Geometry check sheet. Reference: the model listing, model coordinates, mm. Face numbers are marked on the shaded views. A direction names the side the tool comes from. Round coordinates to 2 decimals unless told otherwise and drop trailing zeros. Loops run counter-clockwise (first coordinate to the right, second up) from the corner with the lowest first, then second, coordinate; pieces in that order, holes last. Notation, with made-up numbers: M 41,41.5 L 73,41.5 A24 cw 73,56.5 Z; hole C -4,-30.75 d8. An arc over 180 degrees is marked long. Use one line per item in the form item = value. Start each with the question number.
1. Set-up check for the marked faces 4, 5, 6, 7 and 8: record each of +Z, -Z, +X, -X, +Y, -Y from which the full face is reachable in a straight line by a thin tool's end or side.
2. Cross-section at A-A (z = 27). Record the boundary of the cut face in (x, y), then the cut area to 3 significant figures.
3. Go/stop test with flat-tipped pins: pin 1 (12.5 mm diameter, centred on x = 0, y = -220, fed in from +Z); pin 2 (17.5 mm diameter, centred on x = 136, z = 13, fed in from -Y); pin 3 (6 mm diameter, centred on x = -20, y = -230, fed in from +Z); pin 4 (5 mm diameter, centred on x = 0.5, y = -229.5, fed in from +Z). Record where each tip stops, or that it passes through.
4. Cross-section at C-C (z = 8). Record the boundary of the cut face in (x, y).
5. Material ranges on line 1 (X direction, y = -250, z = 25.25); line 2 (Y direction, x = 0, z = 5.75); line 3 (X direction, y = -252.5, z = 26), recorded low to high.
6. Cross-section at D-D (y = -220). Record the boundary of the cut face in (x, z), then the cut area to 3 significant figures.
7. Cross-section at B-B (y = -250). Record the boundary of the cut face in (x, z).
8. Draft check along X on the marked faces 1, 2 and 3. Enter one of: pulls with the +X half, pulls with the -X half, needs draft (parallel to the pull), parting line crosses it, or undercut.
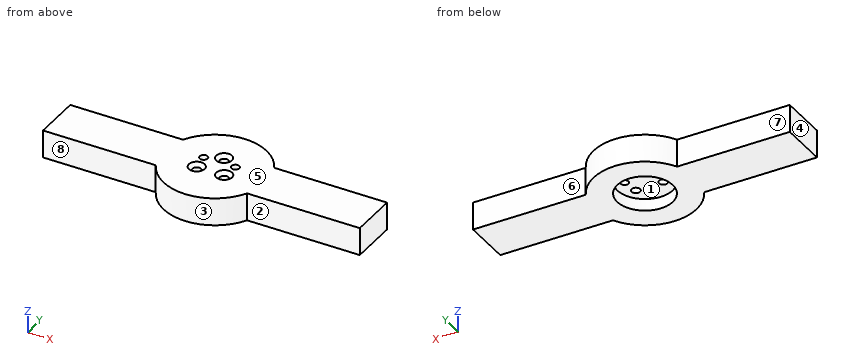
```python
from build123d import *

# Parameters (mm, degrees)
RESSALTO_EXTRUS_O1_DEPTH                             = 35
ESBO_O3_R                                            = 35
CORTE_EXTRUS_O2_DEPTH                                = 15
ESCAREADO_PARA_PARAFUSO_COM_CABE_A_ESCAR_D           = 11
ESCAREADO_PARA_PARAFUSO_COM_CABE_A_ESCAR_CSINK_D     = 20
ESCAREADO_PARA_PARAFUSO_COM_CABE_A_ESCAR_CSINK_ANGLE = 90
FUROS_GUIA_COM_10_0MM1_D                             = 10
ESBO_O2_R                                            = 35
CORTE_EXTRUS_O1_DEPTH                                = 15


with BuildPart() as part:
    # Esboço1 → Ressalto-extrusão1 (new body)
    with BuildSketch(Plane.XY):
        with BuildLine():
            Line((-200, -270), (-57.662812973, -270))
            ThreePointArc((-57.662812973, -270), (0, -305), (57.662812973, -270))
            Line((57.662812973, -270), (200, -270))
            Line((200, -270), (200, -210))
            Line((200, -210), (57.662812973, -210))
            ThreePointArc((57.662812973, -210), (0, -175), (-57.662812973, -210))
            Line((-57.662812973, -210), (-200, -210))
            Line((-200, -210), (-200, -270))
        make_face()
    extrude(amount=RESSALTO_EXTRUS_O1_DEPTH)

    # Esboço3 → Corte-extrusão2 (cut)
    with BuildSketch(Plane(origin=(0, 0, 0), x_dir=(-1, 0, 0), z_dir=(0, 0, -1))):
        with Locations((0, -240)):
            Circle(ESBO_O3_R)
    extrude(amount=-CORTE_EXTRUS_O2_DEPTH, mode=Mode.SUBTRACT)

    # Escareado para parafuso com cabeça escareada elevada de M101 (through all)
    with Locations(Plane.XY.offset(35)):
        with Locations((0, -220), (-17.320508076, -250), (17.320508076, -250)):
            CounterSinkHole(ESCAREADO_PARA_PARAFUSO_COM_CABE_A_ESCAR_D / 2, ESCAREADO_PARA_PARAFUSO_COM_CABE_A_ESCAR_CSINK_D / 2, counter_sink_angle=ESCAREADO_PARA_PARAFUSO_COM_CABE_A_ESCAR_CSINK_ANGLE)

    # Furos-guia com Ø10.0mm1 (through all)
    with Locations(Plane.XY.offset(35)):
        with Locations((-20, -230), (20, -230)):
            Hole(FUROS_GUIA_COM_10_0MM1_D / 2)

    # Esboço2 → Corte-extrusão1 (cut)
    with BuildSketch(Plane(origin=(0, 0, 0), x_dir=(-1, 0, 0), z_dir=(0, 0, -1))):
        with Locations((0, -240)):
            Circle(ESBO_O2_R)
    extrude(amount=-CORTE_EXTRUS_O1_DEPTH, mode=Mode.SUBTRACT)


solid = part.part
```
Reported:
q1.face_4 = +Z, -Z, -X, +Y, -Y
q1.face_5 = +Z, +X, -X, +Y, -Y
q1.face_6 = +Z, -Z, +X, +Y
q1.face_7 = +Z, -Z, -X, +Y
q1.face_8 = +Z, -Z, -X, -Y
q2.outline = M -200,-270 L -57.66,-270 A65 ccw 57.66,-270 L 200,-270 L 200,-210 L 57.66,-210 A65 ccw -57.66,-210 L -200,-210 Z; hole C -20,-230 d10; hole C -17.32,-250 d11; hole C 0,-220 d11; hole C 17.32,-250 d11; hole C 20,-230 d10
q2.area = 29,300 mm²
q3.pin_1 = 31.25
q3.pin_2 = -270
q3.pin_3 = through
q3.pin_4 = 35
q4.outline = M -200,-270 L -57.66,-270 A65 ccw 57.66,-270 L 200,-270 L 200,-210 L 57.66,-210 A65 ccw -57.66,-210 L -200,-210 Z; hole C 0,-240 d70
q5.line_1 = -200 to -22.82, -11.82 to 11.82, 22.82 to 200
q5.line_2 = -305 to -275, -205 to -175
q5.line_3 = -200 to -22.22, -12.42 to 12.42, 22.22 to 200
q6.outline = M -200,0 L -28.72,0 L -28.72,15 L -5.5,15 L -5.5,30.5 L -10,35 L -200,35 Z; M 5.5,15 L 28.72,15 L 28.72,0 L 200,0 L 200,35 L 10,35 L 5.5,30.5 Z
q6.area = 12,900 mm²
q7.outline = M -200,0 L -33.54,0 L -33.54,15 L -22.82,15 L -22.82,30.5 L -27.32,35 L -200,35 Z; M -11.82,15 L 11.82,15 L 11.82,30.5 L 7.32,35 L -7.32,35 L -11.82,30.5 Z; M 22.82,15 L 33.54,15 L 33.54,0 L 200,0 L 200,35 L 27.32,35 L 22.82,30.5 Z
q8.face_1 = undercut
q8.face_2 = needs draft
q8.face_3 = parting line crosses it
